Model file for the job. Use its own axes, mm. Face numbers are marked on the shaded views. Give positions to 0.01 mm unless a question says otherwise; leave off trailing zeros. Loops run counter-clockwise (first coordinate to the right, second up) from the corner with the lowest first, then second, coordinate; pieces in that order, holes last. Notation, with made-up numbers: (4, -6) - (61, -6) arc R16 ccw to (61, -2) - close; hole circle Ø1 at (68, 38). An arc over 180 degrees is marked (long way). Answer as CSV lines item,"result". Start each with the question number.
Item 1: Saw through at A-A on x = 0. Give the cut face in (y, z).
Item 2: Saw through at C-C on z = 1.75. Give the cut face in (x, y), plus the area to 3 significant figures.
Item 3: Drill centre lines: L1, parallel to Y at x = 0, z = 4; L2, parallel to Z at x = -0.5, y = 6; L3, parallel to X at y = 9.25, z = 3. Where is each one in solid material? Low to high. Write a range as from..to.
Item 4: Pull direction Y, two halves, no side cores. Call the marked faces 1, 2 and 3: pulls with the +Y half, pulls with the -Y half, needs draft (parallel to the pull), parting line crosses it, or undercut.
Item 5: Pin check, flat tips, straight feed: pin 1 (1 mm diameter, centred on y = 10, z = 2, fed in from -X); pin 2 (3 mm diameter, centred on y = -4.5, z = 11.5, fed in from -X); pin 3 (5 mm diameter, centred on y = -6.5, z = 15.5, fed in from +X); pin 4 (10 mm diameter, centred on x = -4.5, z = 9.5, fed in from +Y). Stop position of each tip, or through.
Item 6: Saw through at D-D on z = 14.25. Give the cut face in (x, y), plus the area to 3 significant figures.
from build123d import *

# Parameters (mm, degrees)
F0_R     = 13
F1_DEPTH = 20
F2_R     = 11.5
F3_DEPTH = 17
F4_R     = 5


with BuildPart() as f1:
    # F0 (on Top) → F1 (new body)
    with BuildSketch(Plane.XY):
        Circle(F0_R)
    extrude(amount=F1_DEPTH)

    # F2 (on face) → F3 (cut)
    with BuildSketch(Plane(origin=(0, 0, 0), x_dir=(1, 0, 0), z_dir=(0, 0, -1))):
        Circle(F2_R)
    extrude(amount=-F3_DEPTH, mode=Mode.SUBTRACT)

    # F4
    f4_edges = [f1.edges().sort_by_distance(p)[0] for p in [
        (-11.5, 0, 17),
    ]]
    fillet(f4_edges, radius=F4_R)


solid = f1.part
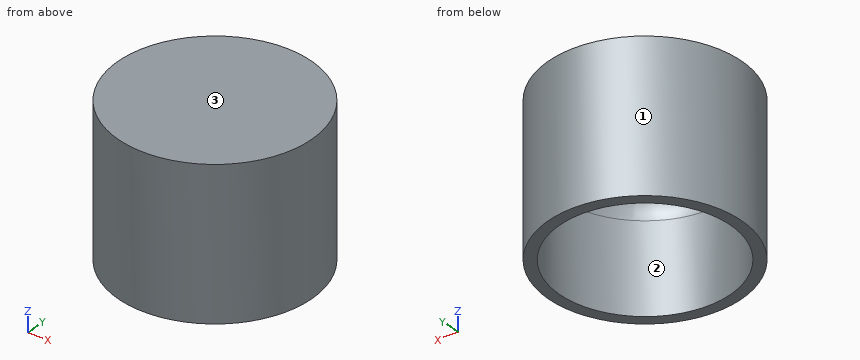
Responses:
1,outline,"(-13, 0) - (-11.5, 0) - (-11.5, 12) arc R5 cw to (-6.5, 17) - (6.5, 17) arc R5 cw to (11.5, 12) - (11.5, 0) - (13, 0) - (13, 20) - (-13, 20) - close"
2,outline,"circle Ø26 at (0, 0); hole circle Ø23 at (0, 0)"
2,area,"115 mm2"
3,L1,"-13..-11.5, 11.5..13"
3,L2,"17..20"
3,L3,"-9.13..-6.83, 6.83..9.13"
4,face 1,"parting line crosses it"
4,face 2,"undercut"
4,face 3,"needs draft"
5,pin 1,"x = -8.87"
5,pin 2,"x = -12.65"
5,pin 3,"x = 12.37"
5,pin 4,"y = 13"
6,outline,"circle Ø26 at (0, 0); hole circle Ø21.93 at (0, 0)"
6,area,"153 mm2"
